Read the model definition and answer for the solid it produces. Units are mm, in the model's axes. Face numbers are marked on the shaded views. Round coordinates to 2 decimals unless told otherwise and drop trailing zeros. Loops run counter-clockwise (first coordinate to the right, second up) from the corner with the lowest first, then second, coordinate; pieces in that order, holes last. Notation, with made-up numbers: (-3.75, 17.5) -> (52.25, 17.5) arc R20 ccw to (52.25, 53.5) -> close; hole circle Ø4 at (88.25, 78.5). An arc over 180 degrees is marked (long way). Put each result on its own line as item: value.
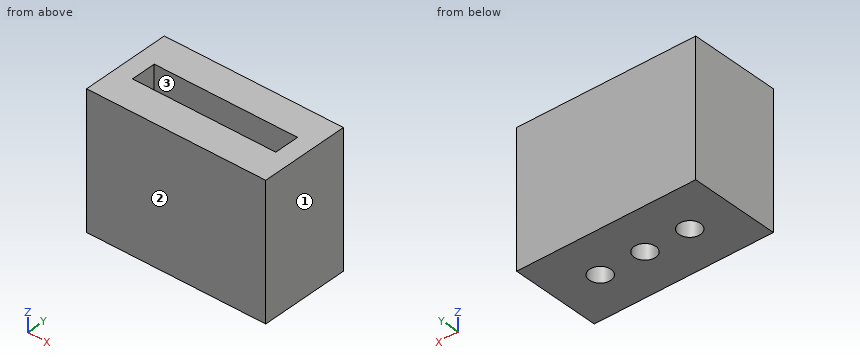
from build123d import *

# Parameters (mm, degrees)
F0_W     = 16
F0_H     = 2.8
F0_R     = 1.2
F1_DEPTH = 2.6
F0_W_2   = 20
F0_H_2   = 10
F2_DEPTH = 15


with BuildPart() as f1:
    # F0 (on Top) → F1 (new body)
    with BuildSketch(Plane.XY):
        with Locations((5, 0)):
            Rectangle(F0_W, F0_H)
        Circle(F0_R, mode=Mode.SUBTRACT)
        with Locations((5, 0)):
            Circle(F0_R, mode=Mode.SUBTRACT)
        with Locations((10, 0)):
            Circle(F0_R, mode=Mode.SUBTRACT)
    extrude(amount=F1_DEPTH)

    # F0 (on Top) → F2 (join)
    with BuildSketch(Plane.XY):
        with Locations((5, 0)):
            Rectangle(F0_W_2, F0_H_2)
        with Locations((5, 0)):
            Rectangle(F0_W, F0_H, mode=Mode.SUBTRACT)
    extrude(amount=F2_DEPTH)


solid = f1.part
Item 1: For a pull along Y with two mould halves and no side action, classify the marked faces 1, 2 and 3 as pulls with the +Y half, pulls with the -Y half, needs draft (parallel to the pull), parting line crosses it, or undercut.
Derived:
face 1: needs draft
face 2: pulls with the -Y half
face 3: undercut
Item 2: The part is cut by section A-A (y = 0). Determine the outline of the cut face in (x, z).
Derived:
outline: (-5, 0) -> (-1.2, 0) -> (-1.2, 2.6) -> (-3, 2.6) -> (-3, 15) -> (-5, 15) -> close; (1.2, 0) -> (3.8, 0) -> (3.8, 2.6) -> (1.2, 2.6) -> close; (6.2, 0) -> (8.8, 0) -> (8.8, 2.6) -> (6.2, 2.6) -> close; (11.2, 0) -> (15, 0) -> (15, 15) -> (13, 15) -> (13, 2.6) -> (11.2, 2.6) -> close
Item 3: A flat-ended cylindrical pin translates along its axis: pin 1 Ø2 at (x, y) = (6, 0) entering from +Z. Find the tip coordinate at first contact, or state that the pin passes through.
Derived:
pin 1: stops at z = 2.6
Item 4: The part is cut by section C-C (x = 5). Determine the outline of the cut face in (y, z).
Derived:
outline: (-5, 0) -> (-1.2, 0) -> (-1.2, 2.6) -> (-1.4, 2.6) -> (-1.4, 15) -> (-5, 15) -> close; (1.2, 0) -> (5, 0) -> (5, 15) -> (1.4, 15) -> (1.4, 2.6) -> (1.2, 2.6) -> close
Item 5: The part is cut by section D-D (z = 1). Determine the outline of the cut face in (x, y).
Derived:
outline: (-5, -5) -> (15, -5) -> (15, 5) -> (-5, 5) -> close; hole circle Ø2.4 at (0, 0); hole circle Ø2.4 at (5, 0); hole circle Ø2.4 at (10, 0)
Item 6: Find the intervals of material crossed by line 1 along X through (y, z) = (0, 6.75); line 2 along Y through (x, z) = (10, 1.5); line 3 along Y through (x, z) = (12.25, 12), in increasing order.
Derived:
line 1: x = -5 to -3, 13 to 15
line 2: y = -5 to -1.2, 1.2 to 5
line 3: y = -5 to -1.4, 1.4 to 5
Item 7: The part is cut by section B-B (z = 3.5). Determine the outline of the cut face in (x, y), then the cut area to 3 significant figures.
Derived:
outline: (-5, -5) -> (15, -5) -> (15, 5) -> (-5, 5) -> close; hole (-3, -1.4) -> (13, -1.4) -> (13, 1.4) -> (-3, 1.4) -> close
area: 155 mm^2
